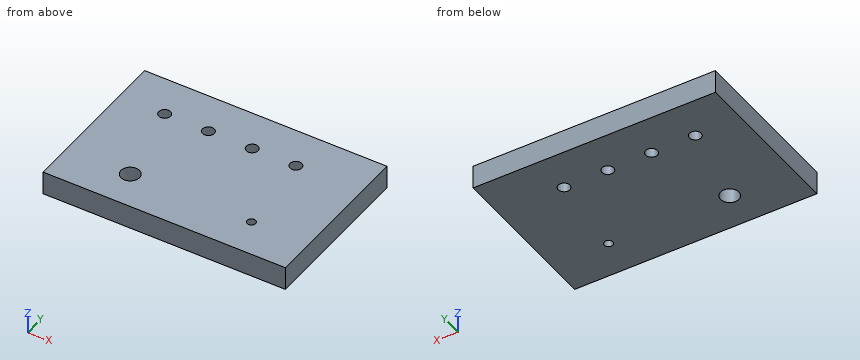
```python
from build123d import *

# Parameters (mm, degrees)
SKETCH_1_W             = 144
SKETCH_1_H             = 96
EXTRUDE_237_DEPTH      = 14
SKETCH_3_R             = 3.5
CUT_EXTRUDE_A_DEPTH    = 88.658428003
PATTERN_LINEAR_2_COUNT = 4
PATTERN_LINEAR_2_PITCH = 26
SKETCH_4_R             = 5.5
CUT_EXTRUDE_B_DEPTH    = 88.658428003
SKETCH_5_R             = 2.5
CUT_EXTRUDE_C_DEPTH    = 88.658428003


with BuildPart() as part:
    # 草图1 → Extrude 237 (new body)
    with BuildSketch(Plane.XY):
        Rectangle(SKETCH_1_W, SKETCH_1_H)
    extrude(amount=EXTRUDE_237_DEPTH)

    # 草图3 → 孔A (cut, through all)
    with BuildSketch(Plane.XY):
        with Locations((-45, 24)):
            Circle(SKETCH_3_R)
    cut_extrude_a = extrude(amount=CUT_EXTRUDE_A_DEPTH, mode=Mode.SUBTRACT)

    # 阵列(线性)2: 孔A ×4
    with Locations(*[(i * PATTERN_LINEAR_2_PITCH, 0, 0) for i in range(1, PATTERN_LINEAR_2_COUNT)]):
        add(cut_extrude_a, mode=Mode.SUBTRACT)

    # 草图4 → 孔B (cut, through all)
    with BuildSketch(Plane.XY):
        with Locations((-34, -26)):
            Circle(SKETCH_4_R)
    extrude(amount=CUT_EXTRUDE_B_DEPTH, mode=Mode.SUBTRACT)

    # 草图5 → 孔C (cut, through all)
    with BuildSketch(Plane.XY):
        with Locations((38, -26)):
            Circle(SKETCH_5_R)
    extrude(amount=CUT_EXTRUDE_C_DEPTH, mode=Mode.SUBTRACT)


solid = part.part
```
Geometry check sheet. Reference: the model listing, model coordinates, mm. Give positions to 0.01 mm unless a question says otherwise; leave off trailing zeros. Order: outer loops, then holes, each group sorted by start corner. A loop starts at its lowest first (then second) coordinate and runs counter-clockwise, first axis right, second up.
1. Gauge pin test, flat end, axial feed: pin 1 Ø9 at (x, y) = (-34, -26) entering from -Z. Record the tip position at first contact, or that the pin passes through.
2. Section check B-B, the plane y = -26. Enter the section's corners in (x, z).
3. Section check C-C, the plane y = 24. Enter the section's corners in (x, z).
4. Thickness scan on L1, parallel to X at y = 24, z = 7.25; L2, parallel to Y at x = -45, z = 3.75; L3, parallel to X at y = 25, z = 2.5. Record the ranges inside material, lowest first.
5. Section check A-A, the plane x = 38. Enter the section's corners in (y, z), and give its area (3 significant figures).
6. Section check D-D, the plane z = 3. Enter the section's corners in (x, y).
Values follow:
1. pin 1: passes through
2. outline: (-72, 0) - (-39.5, 0) - (-39.5, 14) - (-72, 14) - close; (-28.5, 0) - (35.5, 0) - (35.5, 14) - (-28.5, 14) - close; (40.5, 0) - (72, 0) - (72, 14) - (40.5, 14) - close
3. outline: (-72, 0) - (-48.5, 0) - (-48.5, 14) - (-72, 14) - close; (-41.5, 0) - (-22.5, 0) - (-22.5, 14) - (-41.5, 14) - close; (-15.5, 0) - (3.5, 0) - (3.5, 14) - (-15.5, 14) - close; (10.5, 0) - (29.5, 0) - (29.5, 14) - (10.5, 14) - close; (36.5, 0) - (72, 0) - (72, 14) - (36.5, 14) - close
4. L1: x = -72 to -48.5, -41.5 to -22.5, -15.5 to 3.5, 10.5 to 29.5, 36.5 to 72
4. L2: y = -48 to 20.5, 27.5 to 48
4. L3: x = -72 to -48.35, -41.65 to -22.35, -15.65 to 3.65, 10.35 to 29.65, 36.35 to 72
5. outline: (-48, 0) - (-28.5, 0) - (-28.5, 14) - (-48, 14) - close; (-23.5, 0) - (48, 0) - (48, 14) - (-23.5, 14) - close
5. area: 1,270 mm2
6. outline: (-72, -48) - (72, -48) - (72, 48) - (-72, 48) - close; hole circle Ø7 at (-45, 24); hole circle Ø11 at (-34, -26); hole circle Ø7 at (-19, 24); hole circle Ø7 at (7, 24); hole circle Ø7 at (33, 24); hole circle Ø5 at (38, -26)
